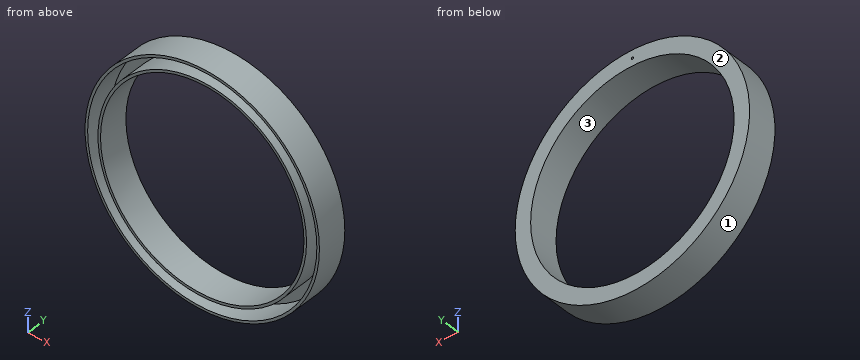
from build123d import *

# Parameters (mm, degrees)
F0_R     = 115.57
F0_R_2   = 100.33
F1_DEPTH = 30
F2_T     = -2.54
F4_D     = 2.1


with BuildPart() as f1:
    # F0 (on Front) → F1 (new body)
    with BuildSketch(Plane.XZ):
        Circle(F0_R)
        Circle(F0_R_2, mode=Mode.SUBTRACT)
    extrude(amount=F1_DEPTH)

    # F2
    f2_openings = [f1.faces().sort_by_distance(p)[0] for p in [
        (-112.301187, -30, 0),
    ]]
    offset(amount=F2_T, openings=f2_openings)

    # F4 (through all)
    with Locations(Plane.XZ.offset(2.54)):
        with Locations((0, 107.667133)):
            Hole(F4_D / 2)


solid = f1.part
The model under review builds one solid part; all positions refer to its coordinate system, in mm. Face numbers are marked on the shaded views. Round coordinates to 2 decimals unless told otherwise and drop trailing zeros. Write each loop counter-clockwise with the first axis right and the second up, starting at its lowest first coordinate (ties: lowest second). Pieces come first, ordered by that corner, then holes. Notation, with made-up numbers: (75, 83) -> (93, 83) arc R25 ccw to (93, 113) -> close; hole circle Ø3 at (25, 49.5). An arc over 180 degrees is marked (long way). Answer as a JSON object with one key per item and string values.
1. The part is to be moulded in two halves that separate along Z. For the marked faces 1, 2 and 3, say which applies: pulls with the +Z half, pulls with the -Z half, needs draft (parallel to the pull), parting line crosses it, or undercut.
Results found:
{"face 1": "parting line crosses it", "face 2": "needs draft", "face 3": "undercut"}
2. Clearance check with flat-ended pins moving along their axes: pin 1 (4 mm diameter, centred on y = -25.5, z = -61.5, fed in from +X); pin 2 (1.5 mm diameter, centred on y = -11.5, z = -61, fed in from -X); pin 3 (6 mm diameter, centred on y = -16.5, z = -77.5, fed in from +X); pin 4 (1.9 mm diameter, centred on x = 0, z = 107.67, fed in from -Y) (3 decimals). State where each tip first meets the part, or that it passes through.
Results found:
{"pin 1": "stops at x = 99.08", "pin 2": "stops at x = -98.62", "pin 3": "stops at x = 88.35", "pin 4": "passes through"}
3. We need section A-A on z = 75. State the section outline as (x, y) points, and give its area (3 significant figures).
Results found:
{"outline": "(-87.93, -30) -> (-84.56, -30) -> (-84.56, -2.54) -> (-70.41, -2.54) -> (-70.41, -30) -> (-66.64, -30) -> (-66.64, 0) -> (-87.93, 0) -> close; (66.64, -30) -> (70.41, -30) -> (70.41, -2.54) -> (84.56, -2.54) -> (84.56, -30) -> (87.93, -30) -> (87.93, 0) -> (66.64, 0) -> close", "area": "500 mm^2"}
4. We need section B-B on x = 45. State the section outline as (y, z) points, and give its area (3 significant figures).
Results found:
{"outline": "(-30, -106.45) -> (0, -106.45) -> (0, -89.67) -> (-30, -89.67) -> (-30, -92.51) -> (-2.54, -92.51) -> (-2.54, -103.69) -> (-30, -103.69) -> close; (-30, 89.67) -> (0, 89.67) -> (0, 106.45) -> (-30, 106.45) -> (-30, 103.69) -> (-2.54, 103.69) -> (-2.54, 92.51) -> (-30, 92.51) -> close", "area": "393 mm^2"}
5. We need section C-C on y = -8. State the section outline as (x, z) points, and give its area (3 significant figures).
Results found:
{"outline": "circle Ø231.14 at (0, 0); circle Ø205.74 at (0, 0); hole circle Ø226.06 at (0, 0); hole circle Ø200.66 at (0, 0)", "area": "3,450 mm^2"}
6. To check wall thickness, follow line 1 along Z through (x, y) = (0, -13.25); line 2 along Z through (x, y) = (0, -0.95); line 3 along X through (y, z) = (-12.75, 54.5). State the ranges of each line that lie inside material, in increasing order.
Results found:
{"line 1": "z = -115.57 to -113.03, -102.87 to -100.33, 100.33 to 102.87, 113.03 to 115.57", "line 2": "z = -115.57 to -100.33, 100.33 to 106.62, 108.72 to 115.57", "line 3": "x = -101.91 to -99.02, -87.25 to -84.24, 84.24 to 87.25, 99.02 to 101.91"}
